```python
from build123d import *
from OCP.BRepFilletAPI import BRepFilletAPI_MakeFillet

# Parameters (mm, degrees)
SKETCH1_R               = 3.175
SKETCH1_R_2             = 1.18999
BOSS_EXTRUDE1_DEPTH     = 0.1905
CUT_EXTRUDE1_DEPTH      = 5.50626353
CUT_EXTRUDE2_DEPTH      = 5.50626353
CUT_EXTRUDE2_DEPTH_BACK = 5.50626353
FILLET1_R1              = 0.127
FILLET1_R2              = 0.381


with BuildPart() as part:
    # Sketch1 → Boss-Extrude1 (new, symmetric)
    with BuildSketch(Plane.XY):
        with Locations(Location((0, 0, 0), (0, 0, 180))):
            Circle(SKETCH1_R)
        with Locations(Location((0, 0, 0), (0, 0, 180))):
            Circle(SKETCH1_R_2, mode=Mode.SUBTRACT)
    extrude(amount=BOSS_EXTRUDE1_DEPTH, both=True)

    # Sketch2 → Cut-Extrude1 (cut, through all)
    with BuildSketch(Plane.XY.offset(0.1905)):
        Polygon((-0.635, 0.3107001), (0.635, 0.3107001), (1.27, 3.175), (-1.27, 3.175), align=None)
    extrude(amount=-CUT_EXTRUDE1_DEPTH, mode=Mode.SUBTRACT)

    # Sketch3 → Cut-Extrude2 (cut, two sides: drawn at the far end of the back side and taken through both)
    with BuildSketch(Plane.XY.offset(0.1905).offset(-CUT_EXTRUDE2_DEPTH_BACK)):
        with BuildLine():
            Line((-1.05664, 0.547346426), (-2.141464207, 1.112070164))
            ThreePointArc((-2.141464207, 1.112070164), (-2.284557926, -0.77676514), (-1.01978636, -2.186916729))
            Line((-1.01978636, -2.186916729), (-0.50292, -1.078493242))
            ThreePointArc((-0.50292, -1.078493242), (-1.12645262, -0.383641362), (-1.05664, 0.547346426))
        make_face()
        with BuildLine():
            Line((0.50292, -1.078493242), (1.01978636, -2.186916729))
            ThreePointArc((1.01978636, -2.186916729), (2.284557926, -0.77676514), (2.141464207, 1.112070164))
            Line((2.141464207, 1.112070164), (1.05664, 0.547346426))
            ThreePointArc((1.05664, 0.547346426), (1.12645262, -0.383641362), (0.50292, -1.078493242))
        make_face()
    extrude(amount=CUT_EXTRUDE2_DEPTH + CUT_EXTRUDE2_DEPTH_BACK, mode=Mode.SUBTRACT)

    # Fillet1: one fillet with a radius per group of edges: ONE call of the kernel's fillet builder (fillet() takes one radius for all edges)
    fillet1_edges_1 = [part.edges().sort_by_distance(p)[0] for p in [
        (-0.929941204, 0.742486065, 0.1905),
        (-0.929941204, 0.742486065, -0.1905),
        (-0.76769373, 0.909242837, 0),
        (0.76769373, 0.909242837, 0),
        (-1.05664, 0.547346426, 0),
        (-1.01978636, -2.186916729, 0),
        (1.05664, 0.547346426, 0),
    ]]
    fillet1_edges_2 = [part.edges().sort_by_distance(p)[0] for p in [
        (1.216302436, 2.932785942, 0),
        (-1.216302436, 2.932785942, 0),
        (-2.141464207, 1.112070164, 0),
        (-0.50292, -1.078493242, 0),
        (1.01978636, -2.186916729, 0),
        (0.50292, -1.078493242, 0),
        (2.141464207, 1.112070164, 0),
    ]]
    fillet1 = BRepFilletAPI_MakeFillet(part.part.solid().wrapped)
    for e in fillet1_edges_1:
        fillet1.Add(FILLET1_R1, e.wrapped)
    for e in fillet1_edges_2:
        fillet1.Add(FILLET1_R2, e.wrapped)
    add(Compound.cast(fillet1.Shape()), mode=Mode.REPLACE)


solid = part.part
```
Work out the finished part from the listing and answer in its coordinate system (mm). A direction names the side the tool comes from. Round coordinates to 2 decimals unless told otherwise and drop trailing zeros. Write each loop counter-clockwise with the first axis right and the second up, starting at its lowest first coordinate (ties: lowest second). Pieces come first, ordered by that corner, then holes. Notation, with made-up numbers: (-24, 61.5) - (9, 61.5) arc R29 ccw to (9, 81.5) - close; hole circle Ø7 at (50.25, -15). An arc over 180 degrees is marked (long way). Return JSON: item names as keys, results as strings. Group by question number.
Q1. Find the intervals of material crossed by L1, parallel to X at y = -0.1, z = -0.05; L2, parallel to X at y = -1.75, z = 0; L3, parallel to X at y = -1.55, z = 0, in increasing order.
Q2. For faces 4 (the flat face through (0, -2, 0.19)), 5 (the cylindrical face through (2.278, -0.797, -0.003)), determine the directions among +Z, -Z, +X, -X, +Y, -Y from which every point of the face is accessible in a straight line to the end or side of a thin tool.
Q3. The mould has two halves that part along X. Classify faces 1 (the cylindrical face through (-2.237, -0.906, -0.003)), 2 (the flat face through (0, -2, -0.19)), 3 (the cylindrical face through (-0.115, -3.173, 0.003)): released by +X, released by -X, zero draft, split by the parting line, or undercut.
Q4. The part is cut by section B-B on x = 1.5. Write down the section's boundary in (y, z), then the cut area to 3 significant figures.
Q5. The part is cut by section C-C on z = 0. Write down the section's boundary in (x, y) (3 decimals), then the cut area to 3 significant figures.
Solved:
{
 "1": {"L1": "-3.17 to -2.41, 2.41 to 3.17", "L2": "-2.65 to -1.66, -0.82 to 0.82, 1.66 to 2.65", "L3": "-2.77 to -1.85, -0.72 to 0.72, 1.85 to 2.77"},
 "2": {"face 4": "+Z, +X, -X, +Y, -Y", "face 5": "+Z, -Z"},
 "3": {"face 1": "undercut", "face 2": "zero draft", "face 3": "split by the parting line"},
 "4": {"outline": "(-2.8, -0.19) - (-1.89, -0.19) - (-1.89, 0.19) - (-2.8, 0.19) - close; (0.78, -0.19) - (2.75, -0.19) - (2.75, 0.19) - (0.78, 0.19) - close", "area": "1.10 mm²"},
 "5": {"outline": "(-2.312, 0.69) arc R0.381 cw to (-1.771, 0.919) - (-1.164, 0.603) arc R0.127 ccw to (-0.999, 0.647) arc R1.19 cw to (-0.82, 0.862) arc R0.127 ccw to (-0.784, 0.982) - (-1.11, 2.451) arc R0.381 ccw to (-1.684, 2.692) arc R3.175 ccw (long way) to (1.684, 2.692) arc R0.381 ccw to (1.11, 2.451) - (0.784, 0.982) arc R0.127 ccw to (0.82, 0.862) arc R1.19 cw to (0.999, 0.647) arc R0.127 ccw to (1.164, 0.603) - (1.771, 0.919) arc R0.381 cw to (2.312, 0.69) arc R2.413 cw to (1.412, -1.957) arc R0.381 cw to (0.844, -1.809) - (0.644, -1.381) arc R0.381 ccw to (0.226, -1.168) arc R1.19 cw to (-0.226, -1.168) arc R0.381 ccw to (-0.644, -1.381) - (-0.965, -2.069) arc R0.127 cw to (-1.14, -2.127) arc R2.413 cw to start", "area": "16.0 mm²"}
}
